Autodesk Inventor part; units mm, degrees
ref_plane "ring_XY" through (0, 0, 0.3937) normal (0, 0, 1) x (1, 0, 0)
ref_plane "ring_YZ" through (0, 0, 0.3937) normal (1, 0, 0) x (0, 1, 0)
ref_plane "ring_ZX" through (0, 0, 0.3937) normal (0, 1, 0) x (0, 0, 1)
sketch "Sketch_4" plane through (0, 0, 0) normal (0, 0, 1) x (1, 0, 0)
  arc A0 (-5.7658, -1.6396) -> (-5.7658, 1.6396) centre (0, 0) ccw
  line L0 (-5.7658, 1.6396) -> (-5.7658, -1.6396)
  line L1 (-3.1648, 0.254) -> (-2.6416, 0.254)
  line L2 (-2.6416, 0.254) -> (-2.6416, -0.254)
  line L3 (-2.6416, -0.254) -> (-3.1648, -0.254)
  arc A1 (-3.1648, -0.254) -> (-3.1648, 0.254) centre (0, 0) ccw
extrude "Extrusion1" add sketch "Sketch_4" along normal blind 0.7874
sketch "Sketch_2" plane through (0, 0, 0) normal (0, 1, 0) x (-1, 0, 0)
  line L0 (6.35, 1.7018) -> (5.7658, 1.7018)
  line L1 (5.7658, 1.7018) -> (5.7658, 0.7874)
  line L2 (5.7658, 0.7874) -> (4.4069, 0.7874)
  line L3 (4.4069, 0.7874) -> (4.4069, 0)
  line L4 (4.4069, 0) -> (5.9563, 0)
  arc A0 (5.9563, 0) -> (6.35, 0.3937) centre (5.9563, 0.3937) ccw
  line L5 (6.35, 0.3937) -> (6.35, 1.7018)
extrude "Extrusion2" add sketch "Sketch_2" along normal mid plane 2.0066
ref_plane "ring_XY" through (0, 0, 0.3937) normal (0, 0, 1) x (1, 0, 0)
ref_plane "ring_YZ" through (0, 0, 0.3937) normal (1, 0, 0) x (0, 1, 0)
ref_plane "ring_ZX" through (0, 0, 0.3937) normal (0, 1, 0) x (0, 0, 1)
properties part number "AT507H"
Verification items for the finished model (mm, model axes). A direction names the side the tool comes from. Coordinates: 2 decimals unless noted, no trailing zeros. Order: outer loops, then holes, each group sorted by start corner. A loop starts at its lowest first (then second) coordinate and runs counter-clockwise, first axis right, second up. Notation, with made-up numbers: (64.5, -35.5) -> (113.5, -35.5) arc R12 cw to (113.5, -25.5) -> close; hole circle Ø11 at (31, 71). An arc over 180 degrees is marked (long way). Put each result on its own line as item: value. Start each with the question number.
1) Cross-section at A-A (x = 0). Enter the section's corners in (y, z), plus the area to 3 significant figures.
2) Material ranges on L1, parallel to X at y = 0, z = 0.65; L2, parallel to Y at x = 0, z = 0.4; L3, parallel to Z at x = -2, y = 5, recorded low to high.
3) Go/stop test with flat-tipped pins: pin 1 (1.5 mm diameter, centred on x = 1, y = -3.5, fed in from +Z); pin 2 (0.6 mm diameter, centred on x = -3, z = 0.5, fed in from -Y); pin 3 (0.7 mm diameter, centred on y = -1.5, z = 0.5, fed in from -X). Record where each tip stops, or that it passes through.
4) Cross-section at C-C (z = 0.6). Enter the section's corners in (x, y).
5) Cross-section at D-D (x = -2.25). Enter the section's corners in (y, z).
6) Release check for a two-part mould opening along X. For faces 3 (the flat face through (-3, 0, 0)), 4 (the cylindrical face through (3.17, 0.14, 0.39)), 5 (the flat face through (-6.35, 0, 1)) record: pulls with the +X half, pulls with the -X half, needs draft (parallel to the pull), parting line crosses it, or undercut.
7) Tool access check on faces 1 (the cylindrical face through (5.99, 0.24, 0.39)), 2 (the flat face through (-5.766, 0, 1)). Record the directions out of +Z, -Z, +X, -X, +Y, -Y that give a thin tool (end or side, any length) a straight path to the whole face; none if there is none.
8) Cross-section at B-B (y = 0). Enter the section's corners in (x, z), plus the area to 3 significant figures.
Geometry check:
1. outline: (-5.99, 0) -> (-3.17, 0) -> (-3.17, 0.79) -> (-5.99, 0.79) -> close; (3.17, 0) -> (5.99, 0) -> (5.99, 0.79) -> (3.17, 0.79) -> close
1. area: 4.44 mm^2
2. L1: x = -6.35 to -2.64, 3.17 to 5.99
2. L2: y = -5.99 to -3.17, 3.17 to 5.99
2. L3: z = 0 to 0.79
3. pin 1: stops at z = 0.79
3. pin 2: stops at y = -5.35
3. pin 3: stops at x = -5.77
4. outline: (-6.35, -1) -> (-5.77, -1) -> (-5.77, -1.64) arc R5.99 ccw (long way) to (-5.77, 1.64) -> (-5.77, 1) -> (-6.35, 1) -> close; hole (-3.16, -0.25) arc R3.17 ccw (long way) to (-3.16, 0.25) -> (-2.64, 0.25) -> (-2.64, -0.25) -> close
5. outline: (-5.56, 0) -> (-2.24, 0) -> (-2.24, 0.79) -> (-5.56, 0.79) -> close; (2.24, 0) -> (5.56, 0) -> (5.56, 0.79) -> (2.24, 0.79) -> close
6. face 3: needs draft
6. face 4: undercut
6. face 5: pulls with the -X half
7. face 1: +Z, -Z
7. face 2: +Z, +X, +Y, -Y
8. outline: (-6.35, 0.39) arc R0.39 ccw to (-5.96, 0) -> (-2.64, 0) -> (-2.64, 0.79) -> (-5.77, 0.79) -> (-5.77, 1.7) -> (-6.35, 1.7) -> close; (3.17, 0) -> (5.99, 0) -> (5.99, 0.79) -> (3.17, 0.79) -> close
8. area: 5.64 mm^2
